from build123d import *


with BuildPart() as part:
    # Sketch2 → Revolve-Thin2 (revolve)
    with BuildSketch(Plane.XY, mode=Mode.PRIVATE) as revolve_thin2_sk:
        Polygon((-150, 0), (-150, 10), (-70, 10), (-70, 30), (-30, 30), (-30, 50), (30, 50), (30, 30), (70, 30), (70, 10), (150, 10), (150, 0), (160, 0), (160, 20), (80, 20), (80, 40), (40, 40), (40, 60), (-40, 60), (-40, 40), (-80, 40), (-80, 20), (-160, 20), (-160, 0), align=None)
    revolve(revolve_thin2_sk.sketch.rotate(Axis((-150, 0, 0), (1, 0, 0)), 90), axis=Axis((-150, 0, 0), (1, 0, 0)))  # turned: the seam where the file's is


solid = part.part
The model under review builds one solid part; all positions refer to its coordinate system, in mm. A direction names the side the tool comes from. Round coordinates to 2 decimals unless told otherwise and drop trailing zeros. Order: outer loops, then holes, each group sorted by start corner. A loop starts at its lowest first (then second) coordinate and runs counter-clockwise, first axis right, second up. Notation, with made-up numbers: (65, 50) -> (115, 50) arc R21 ccw to (115, 63) -> close; hole circle Ø10 at (47.25, -1.5). An arc over 180 degrees is marked (long way). Return JSON: item names as keys, results as strings.
1. The part is to be moulded in two halves that separate along Y. For faces 4 (the face through (-0.56, -50.59, 32.26)), 5 (the face through (80, -18.3, 9.4)), 6 (the face through (-70, 0, -13)), say which applies: +Y half, -Y half, draft (parallel to the pull), parting line (faces both ways), or undercut.
Answer block:
{"face 4": "parting line", "face 5": "draft", "face 6": "undercut"}
2. For L1, parallel to X at y = -15, z = -20; L2, parallel to X at y = 16.5, z = 28.5; L3, parallel to Y at x = -22, z = 0.5, list the stretches that pass through material, from the lowest coordinate up. Write a range as [from, to].
Answer block:
{"L1": "x = [-80, -70], [70, 80]", "L2": "x = [-80, -30], [30, 80]", "L3": "y = [-60, -50], [50, 60]"}
3. Take a section at A-A (x = -86). Write out the cut boundary in (y, z).
Answer block:
{"outline": "circle Ø40 at (0, 0); hole circle Ø20 at (0, 0)"}
4. Take a section at B-B (y = -37). Write out the cut boundary in (x, z), then the cut area to 3 significant figures.
Answer block:
{"outline": "(-80, -15.2) -> (-40, -15.2) -> (-40, -47.23) -> (40, -47.23) -> (40, -15.2) -> (80, -15.2) -> (80, 15.2) -> (40, 15.2) -> (40, 47.23) -> (-40, 47.23) -> (-40, 15.2) -> (-80, 15.2) -> close; hole (-30, -33.63) -> (30, -33.63) -> (30, 33.63) -> (-30, 33.63) -> close", "area": "5,950 mm²"}
5. For faces 1 (the face through (-109, 0, -10)), 2 (the face through (59.72, -1.76, -39.96)), 3 (the face through (-40, 39, 12)), list the 3-axis set-ups (+Z, -Z, +X, -X, +Y, -Y) from which the entire face can be reached by the end or side of a thin tool; tool diameter is ignored.
Answer block:
{"face 1": "none", "face 2": "+X", "face 3": "-X"}
6. Insertion check: P1, Ø6, axis at x = -26, y = 5, coming from the -Z side; P2, Ø10, axis at y = 4, z = 26.5, coming from the -X side; P3, Ø4, axis at x = 117.5, z = 3, coming from the +Y side (3 decimals). Each pin has a flat end and moves straight along its axis. Give the tip position at first contact, or say it passes through.
Answer block:
{"P1": "stops at z = -59.97", "P2": "stops at x = -80", "P3": "stops at y = 19.975"}
